The listing builds one solid part. Answer for the finished solid, in the listing's coordinates (mm). A direction names the side the tool comes from. Round coordinates to 2 decimals unless told otherwise and drop trailing zeros. Order: outer loops, then holes, each group sorted by start corner. A loop starts at its lowest first (then second) coordinate and runs counter-clockwise, first axis right, second up. Notation, with made-up numbers: (43, 2.25) - (102, 2.25) arc R22 cw to (102, 33.25) - close; hole circle Ø3 at (65, 88). An arc over 180 degrees is marked (long way). One line per item, written item: value. Start each with the question number.
1. Flat-ended cylindrical pins translate along their axes: P1, Ø9.5, axis at x = 50.86, y = -52.5, coming from the -Z side (1 decimal); P2, Ø11.5, axis at x = -52.03, y = 56.55, coming from the +Z side; P3, Ø5, axis at x = 23.5, z = 78.5, coming from the -Y side; P4, Ø1.5, axis at y = 22.5, z = 43, coming from the +X side. Find the tip coordinate at first contact, or state that the pin passes through.
2. Straight lines are drawn through the part: line 1 (Y direction, x = 53.5, z = 23.5); line 2 (Z direction, x = 0.5, y = 42.5); line 3 (X direction, y = 3, z = 37). For each, find the intervals that lie inside material, in ascending order.
3. Section A-A, the plane y = 0 is taken. Give the vertices of the cut face in (x, z), then the cut area to 3 significant figures.
4. For a pull along Z with two mould halves and no side action, classify faces 4 (the cylindrical face through (47.111, 59.987, 12.878)), 5 (the flat face through (21, 9, 63.5)), 6 (the flat face through (0.233, -61.62, 22.824)), 7 (the flat face through (0, 3, 0)) as released by +Z, released by -Z, zero draft, split by the parting line, or undercut.
5. A tool of negligible diameter and unlimited length cuts with its end or side. For faces 1 (the flat face through (0, 0, 88.9)), 2 (the flat face through (21, -9, 50.8)), 3 (the cylindrical face through (-6.28, -28.27, 35.42)), from which of +Z, -Z, +X, -X, +Y, -Y can it reach the whole face along a straight path? Write none if from no direction.
6. Section C-C, the plane z = 38 is taken. Give the vertices of the cut face in (x, y).
7. Section D-D, the plane x = 0 is taken. Give the vertices of the cut face in (y, z).
8. Section B-B, the plane x = -33 is taken. Give the vertices of the cut face in (y, z).
from build123d import *

# Parameters (mm, degrees)
F0_W      = 133.204266
F0_H      = 132.038363
F1_DEPTH  = 25.4
F2_R      = 5.014733
F2_R_2    = 5.090399
F2_R_3    = 5.903397
F2_R_4    = 5.940857
F4_DEPTH  = 25.4
F5_DEPTH  = 25.4
F3_R      = 28.959294
F6_DEPTH  = 25.4
F7_R      = 22.678724
F8_DEPTH  = 12.7
F9_R      = 28.767789
F10_DEPTH = 25.4
F11_R     = 5.08
F12_SIZE  = 5.08


with BuildPart() as f1:
    # F0 (on Top) → F1 (new body)
    with BuildSketch(Plane.XY):
        with Locations((1.165904, 1.89459)):
            Rectangle(F0_W, F0_H)
    extrude(amount=F1_DEPTH)

    # F2 (on face) → F4 (cut)
    with BuildSketch(Plane.XY.offset(25.4)):
        with Locations((-52.031644, 56.54623)):
            Circle(F2_R)
        with Locations((50.862458, 56.54623)):
            Circle(F2_R_2)
        with Locations((-52.031644, -51.589914)):
            Circle(F2_R_3)
        with Locations((50.862458, -52.49856)):
            Circle(F2_R_4)
    extrude(amount=-F4_DEPTH, mode=Mode.SUBTRACT)

    # F2 (on face) → F5 (cut)
    with BuildSketch(Plane.XY.offset(25.4)):
        with Locations((-52.031644, 56.54623)):
            Circle(F2_R)
        with Locations((50.862458, 56.54623)):
            Circle(F2_R_2)
        with Locations((-52.031644, -51.589914)):
            Circle(F2_R_3)
        with Locations((50.862458, -52.49856)):
            Circle(F2_R_4)
    extrude(amount=-F5_DEPTH, mode=Mode.SUBTRACT)

    # F3 (on face) → F6 (join)
    with BuildSketch(Plane.XY.offset(25.4)):
        Circle(F3_R)
    extrude(amount=F6_DEPTH)

    # F7 (on face) → F8 (join)
    with BuildSketch(Plane.XY.offset(50.8)):
        Circle(F7_R)
    extrude(amount=F8_DEPTH)

    # F9 (on face) → F10 (join)
    with BuildSketch(Plane.XY.offset(63.5)):
        Circle(F9_R)
    extrude(amount=F10_DEPTH)

    # F11
    f11_edges = [f1.edges().sort_by_distance(p)[0] for p in [
        (-28.959294, 0, 50.8),
        (-28.767789, 0, 88.9),
    ]]
    fillet(f11_edges, radius=F11_R)

    # F12
    f12_edges = [f1.edges().sort_by_distance(p)[0] for p in [
        (1.165904, -64.124592, 25.4),
        (-65.436229, 1.89459, 25.4),
        (1.165904, 67.913771, 25.4),
        (67.768037, 1.89459, 25.4),
    ]]
    chamfer(f12_edges, length=F12_SIZE)


solid = f1.part
Answer list:
1. P1: passes through
1. P2: stops at z = 25.4
1. P3: stops at y = -19.66
1. P4: stops at x = 19.12
2. line 1: y = -60.94 to -57.82, -47.18 to 52.19, 60.9 to 64.73
2. line 2: z = 0 to 25.4
2. line 3: x = -28.8 to 28.8
3. outline: (-65.44, 0) - (67.77, 0) - (67.77, 20.32) - (62.69, 25.4) - (28.96, 25.4) - (28.96, 45.72) arc R5.08 ccw to (23.88, 50.8) - (22.68, 50.8) - (22.68, 63.5) - (28.77, 63.5) - (28.77, 83.82) arc R5.08 ccw to (23.69, 88.9) - (-23.69, 88.9) arc R5.08 ccw to (-28.77, 83.82) - (-28.77, 63.5) - (-22.68, 63.5) - (-22.68, 50.8) - (-23.88, 50.8) arc R5.08 ccw to (-28.96, 45.72) - (-28.96, 25.4) - (-60.36, 25.4) - (-65.44, 20.32) - close
3. area: 6,840 mm²
4. face 4: zero draft
4. face 5: undercut
4. face 6: released by +Z
4. face 7: released by -Z
5. face 1: +Z, +X, -X, +Y, -Y
5. face 2: none
5. face 3: +Z
6. outline: circle Ø57.92 at (0, 0)
7. outline: (-64.12, 0) - (67.91, 0) - (67.91, 20.32) - (62.83, 25.4) - (28.96, 25.4) - (28.96, 45.72) arc R5.08 ccw to (23.88, 50.8) - (22.68, 50.8) - (22.68, 63.5) - (28.77, 63.5) - (28.77, 83.82) arc R5.08 ccw to (23.69, 88.9) - (-23.69, 88.9) arc R5.08 ccw to (-28.77, 83.82) - (-28.77, 63.5) - (-22.68, 63.5) - (-22.68, 50.8) - (-23.88, 50.8) arc R5.08 ccw to (-28.96, 45.72) - (-28.96, 25.4) - (-59.04, 25.4) - (-64.12, 20.32) - close
8. outline: (-64.12, 0) - (67.91, 0) - (67.91, 20.32) - (62.83, 25.4) - (-59.04, 25.4) - (-64.12, 20.32) - close
